For this review, take the finished solid that the model builds, in its own axes (mm). Face numbers are marked on the shaded views. A direction names the side the tool comes from. Give positions to 0.01 mm unless a question says otherwise; leave off trailing zeros. Order: outer loops, then holes, each group sorted by start corner. A loop starts at its lowest first (then second) coordinate and runs counter-clockwise, first axis right, second up. Notation, with made-up numbers: M 68.5,32 L 122.5,32 A28 ccw 122.5,56 Z; hole C -8,-8.5 d1. An arc over 180 degrees is marked long. Answer as CSV lines item,"result". Start each with the question number.
1. We need section B-B, the plane y = 11.5. Give the boundary of the cut face in (x, z).
2. For line 1 along X through (y, z) = (5, 18.5); line 2 along X through (y, z) = (58.5, 16.5); line 3 along Y through (x, z) = (-5, 8.75), list the stretches that pass through material, from the lowest coordinate up.
3. We need section A-A, the plane z = 20.25. Give the boundary of the cut face in (x, y), and give its area (3 significant figures).
4. Machinability: for the marked faces 4, 5 and 6, which of the approach directions +Z, -Z, +X, -X, +Y, -Y give a long, thin tool a straight path to every point of the face, cutting with its end or side? Answer none if there is none.
5. We need section C-C, the plane x = -31. Give the boundary of the cut face in (y, z).
6. We need section D-D, the plane x = 10. Give the boundary of the cut face in (y, z), and give its area (3 significant figures).
7. Mouldability with a two-part tool opening along Y and no side actions: class the marked faces 1, 2 and 3 as pulls with the +Y half, pulls with the -Y half, needs draft (parallel to the pull), parting line crosses it, or undercut.
8. Clearance check with flat-ended pins moving along their axes: P1, Ø1.5, axis at y = 39.5, z = 19.5, coming from the +X side; P2, Ø9, axis at y = 39.5, z = 15.5, coming from the -X side; P3, Ø12, axis at x = -22.5, z = 5, coming from the -Y side. State where each tip first meets the part, or that it passes through.
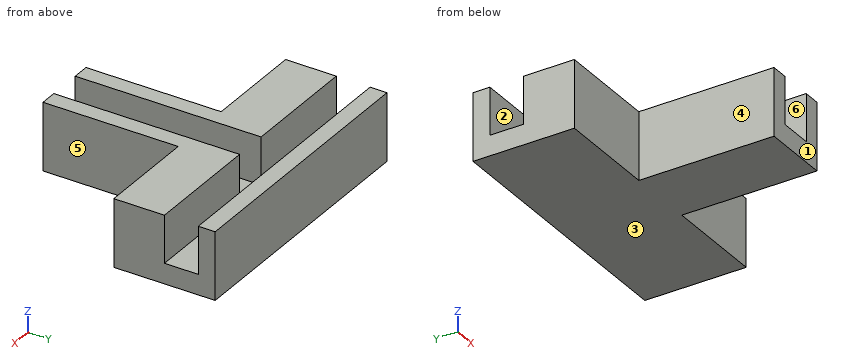
from build123d import *

# Parameters (mm, degrees)
F0_W     = 25.4
F0_H     = 50.8
F0_W_2   = 38.1
F0_H_2   = 38.1
F1_DEPTH = 25.4
F2_W     = 12.7
F2_H     = 19.05
F2_H_2   = 50.8
F3_DEPTH = 17.78


with BuildPart() as f1:
    # F0 (on Top) → F1 (new body)
    with BuildSketch(Plane.XY):
        with Locations((12.7, 25.4)):
            Rectangle(F0_W, F0_H)
        with Locations((44.45, 69.85)):
            Rectangle(F0_W_2, F0_H_2)
        with Locations((12.7, 69.85)):
            Rectangle(F0_W, F0_H_2)
        with Locations((-19.05, 69.85)):
            Rectangle(F0_W_2, F0_H_2)
    extrude(amount=F1_DEPTH)

    # F2 (on face) → F3 (cut)
    with BuildSketch(Plane.XY.offset(25.4)):
        Polygon((-38.1, 69.85), (6.35, 69.85), (19.05, 69.85), (63.5, 69.85), (63.5, 82.55), (-38.1, 82.55), align=None)
        with Locations((12.7, 60.325)):
            Rectangle(F2_W, F2_H)
        with Locations((12.7, 25.4)):
            Rectangle(F2_W, F2_H_2)
    extrude(amount=-F3_DEPTH, mode=Mode.SUBTRACT)


solid = f1.part
Result set:
1,outline,"M 0,0 L 25.4,0 L 25.4,25.4 L 19.05,25.4 L 19.05,7.62 L 6.35,7.62 L 6.35,25.4 L 0,25.4 Z"
2,line 1,"0 to 6.35, 19.05 to 25.4"
2,line 2,"-38.1 to 6.35, 19.05 to 63.5"
2,line 3,"50.8 to 69.85, 82.55 to 88.9"
3,outline,"M -38.1,50.8 L 0,50.8 L 0,0 L 6.35,0 L 6.35,69.85 L -38.1,69.85 Z; M -38.1,82.55 L 63.5,82.55 L 63.5,88.9 L -38.1,88.9 Z; M 19.05,0 L 25.4,0 L 25.4,50.8 L 63.5,50.8 L 63.5,69.85 L 19.05,69.85 Z"
3,area,"2,980 mm2"
4,face 4,"+Z, -Z, -X, -Y"
4,face 5,"+Z, -Z, +X, -Y"
4,face 6,"+Z, -Y"
5,outline,"M 50.8,0 L 88.9,0 L 88.9,25.4 L 82.55,25.4 L 82.55,7.62 L 69.85,7.62 L 69.85,25.4 L 50.8,25.4 Z"
6,outline,"M 0,0 L 88.9,0 L 88.9,25.4 L 82.55,25.4 L 82.55,7.62 L 0,7.62 Z"
6,area,"790 mm2"
7,face 1,"pulls with the -Y half"
7,face 2,"undercut"
7,face 3,"needs draft"
8,P1,"x = 25.4"
8,P2,"x = 0"
8,P3,"y = 50.8"
